from build123d import *

# Parameters (mm, degrees)
IZIM1_W                     = 140
IZIM1_H                     = 65
Y_KSEKLIK_EKSTR_ZYON1_DEPTH = 25
BO_ALTMA3_T                 = 6
IZIM2_R                     = 2.25
KES_EKSTR_ZYON1_DEPTH       = 25
IZIM3_W                     = 13.33242511
IZIM3_H                     = 17.74072696
KES_EKSTR_ZYON2_DEPTH       = 25
RADYUS1_R                   = 2
IZIM2_2_R                   = 2.25
Y_KSEKLIK_EKSTR_ZYON2_DEPTH = 56
IZIM4_W                     = 373.647540747
IZIM4_H                     = 192.392001967
KES_EKSTR_ZYON3_DEPTH       = 1
IZIM5_R                     = 2.25
KES_EKSTR_ZYON4_DEPTH       = 25
IZIM6_W                     = 175.161164464
IZIM6_H                     = 86.760539326
KES_EKSTR_ZYON5_DEPTH       = 37
IZIM7_R                     = 2.25
Y_KSEKLIK_EKSTR_ZYON3_DEPTH = 30
IZIM8_R                     = 1
KES_EKSTR_ZYON6_DEPTH       = 16
KES_EKSTR_ZYON7_START       = -16
IZIM9_R                     = 1
KES_EKSTR_ZYON7_DEPTH       = 16
M2_DI_LI_DELIK2_D           = 1.6
M2_DI_LI_DELIK2_CSINK_D     = 2.05
M2_DI_LI_DELIK2_CSINK_ANGLE = 82
M2_DI_LI_DELIK3_D           = 1.6
M2_DI_LI_DELIK3_CSINK_D     = 2.05
M2_DI_LI_DELIK3_CSINK_ANGLE = 82
IZIM16_W                    = 12
IZIM16_H                    = 6
IZIM16_R                    = 1
Y_KSEKLIK_EKSTR_ZYON4_DEPTH = 2.5
Y_KSEKLIK_EKSTR_ZYON5_START = 2.5
IZIM17_W                    = 12
IZIM17_H                    = 6
IZIM17_R                    = 1
Y_KSEKLIK_EKSTR_ZYON5_DEPTH = 2.5
PAH1_SIZE                   = 2.5


# Read off the part's stored shape, not the designer's step: M2 Dişli Delik4
with BuildPart() as part:
    # Çizim1 → Yükseklik-Ekstrüzyon1 (new body)
    with BuildSketch(Plane.XY):
        Rectangle(IZIM1_W, IZIM1_H)
    extrude(amount=Y_KSEKLIK_EKSTR_ZYON1_DEPTH)

    # İç Boşaltma3
    bo_altma3_openings = [part.faces().sort_by_distance(p)[0] for p in [
        (0, 0, 0),
    ]]
    offset(amount=BO_ALTMA3_T, openings=bo_altma3_openings, kind=Kind.INTERSECTION)

    # Çizim2 → Kes-Ekstrüzyon1 (cut)
    with BuildSketch(Plane(origin=(0, 0, 0), x_dir=(-1, 0, 0), z_dir=(0, 0, -1))):
        with Locations((-73, -35.5)):
            Circle(IZIM2_R)
        with Locations(Location((73, -35.5, 0), (0, 0, 180))):
            Circle(IZIM2_R)
        with Locations(Location((-73, 35.5, 0), (0, 0, 180))):
            Circle(IZIM2_R)
        with Locations((73, 35.5)):
            Circle(IZIM2_R)
    extrude(amount=-KES_EKSTR_ZYON1_DEPTH, mode=Mode.SUBTRACT)

    # Çizim3 → Kes-Ekstrüzyon2 (cut)
    with BuildSketch(Plane.ZY.offset(-70)):
        with Locations((15.822558672, 0)):
            Rectangle(IZIM3_W, IZIM3_H)
    extrude(amount=-KES_EKSTR_ZYON2_DEPTH, mode=Mode.SUBTRACT)

    # Radyus1
    radyus1_edges = [part.edges().sort_by_distance(p)[0] for p in [
        (76, -38.5, 15.5),
        (-76, -38.5, 15.5),
        (-76, 38.5, 15.5),
        (76, 38.5, 15.5),
    ]]
    fillet(radyus1_edges, radius=RADYUS1_R)

    # Çizim2<2> → Yükseklik-Ekstrüzyon2 (add)
    with BuildSketch(Plane(origin=(0, 0, 0), x_dir=(-1, 0, 0), z_dir=(0, 0, -1))):
        with Locations((-73, -35.5)):
            Circle(IZIM2_2_R)
        with Locations((73, -35.5)):
            Circle(IZIM2_2_R)
        with Locations((-73, 35.5)):
            Circle(IZIM2_2_R)
        with Locations((73, 35.5)):
            Circle(IZIM2_2_R)
    extrude(amount=-Y_KSEKLIK_EKSTR_ZYON2_DEPTH)

    # Çizim4 → Kes-Ekstrüzyon3 (cut)
    with BuildSketch(Plane.XY.offset(56)):
        with Locations((-92.221826013, 44.195860188)):
            Rectangle(IZIM4_W, IZIM4_H)
    extrude(amount=-KES_EKSTR_ZYON3_DEPTH, mode=Mode.SUBTRACT)

    # Çizim5 → Kes-Ekstrüzyon4 (cut)
    with BuildSketch(Plane(origin=(0, 0, 0), x_dir=(-1, 0, 0), z_dir=(0, 0, -1))):
        with Locations((-73, -35.527793561)):
            Circle(IZIM5_R)
        with Locations(Location((-73, 35.527793561, 0), (0, 0, 180))):
            Circle(IZIM5_R)
        with Locations((73, 35.527793561)):
            Circle(IZIM5_R)
        with Locations(Location((73, -35.527793561, 0), (0, 0, 180))):
            Circle(IZIM5_R)
    extrude(amount=-KES_EKSTR_ZYON4_DEPTH, mode=Mode.SUBTRACT)

    # Çizim6 → Kes-Ekstrüzyon5 (cut)
    with BuildSketch(Plane.XY.offset(31)):
        Rectangle(IZIM6_W, IZIM6_H)
    extrude(amount=KES_EKSTR_ZYON5_DEPTH, mode=Mode.SUBTRACT)

    # Çizim7 → Yükseklik-Ekstrüzyon3 (add)
    with BuildSketch(Plane(origin=(0, 0, 0), x_dir=(-1, 0, 0), z_dir=(0, 0, -1))):
        with Locations((-73, 35.527793561)):
            Circle(IZIM7_R)
        with Locations((-73, -35.527793561)):
            Circle(IZIM7_R)
        with Locations((73, -35.527793561)):
            Circle(IZIM7_R)
        with Locations((73, 35.527793561)):
            Circle(IZIM7_R)
    extrude(amount=-Y_KSEKLIK_EKSTR_ZYON3_DEPTH)

    # Çizim8 → Kes-Ekstrüzyon6 (cut)
    with BuildSketch(Plane(origin=(76, 0, 0), x_dir=(0, 0, -1), z_dir=(1, 0, 0))):
        with Locations((-3, 28.5)):
            Circle(IZIM8_R)
        with Locations(Location((-3, -28.5, 0), (0, 0, 180))):
            Circle(IZIM8_R)
    extrude(amount=-KES_EKSTR_ZYON6_DEPTH, mode=Mode.SUBTRACT)

    # Çizim9 → Kes-Ekstrüzyon7 (cut)
    with BuildSketch(Plane.ZY.offset(76).offset(KES_EKSTR_ZYON7_START)):
        with Locations(Location((3, 28.5, 0), (0, 0, 180))):
            Circle(IZIM9_R)
        with Locations((3, -28.5)):
            Circle(IZIM9_R)
    extrude(amount=KES_EKSTR_ZYON7_DEPTH, mode=Mode.SUBTRACT)

    # M2 Dişli Delik2 (through all)
    with Locations(Plane(origin=(-76, 28.5, 3), x_dir=(0, 0, -1), z_dir=(-1, 0, 0))):
        with Locations((0, 0), (0, 57)):
            CounterSinkHole(M2_DI_LI_DELIK2_D / 2, M2_DI_LI_DELIK2_CSINK_D / 2, counter_sink_angle=M2_DI_LI_DELIK2_CSINK_ANGLE)

    # M2 Dişli Delik3 (through all)
    with Locations(Plane(origin=(76, 28.5, 3), x_dir=(0, 0, 1), z_dir=(1, 0, 0))):
        with Locations((0, 0), (0, 57)):
            CounterSinkHole(M2_DI_LI_DELIK3_D / 2, M2_DI_LI_DELIK3_CSINK_D / 2, counter_sink_angle=M2_DI_LI_DELIK3_CSINK_ANGLE)

    # Çizim16 → Yükseklik-Ekstrüzyon4 (add)
    # profile 1 of 2: a face of its own
    with BuildSketch(Plane(origin=(76, 0, 0), x_dir=(0, 0, -1), z_dir=(1, 0, 0))):
        with Locations((-31, 28.5)):
            Rectangle(IZIM16_W, IZIM16_H)
        with Locations((-34, 28.5)):
            Circle(IZIM16_R, mode=Mode.SUBTRACT)
    # profile 2 of 2: a face of its own
    with BuildSketch(Plane(origin=(76, 0, 0), x_dir=(0, 0, -1), z_dir=(1, 0, 0))):
        with Locations((-31, -28.5)):
            Rectangle(IZIM16_W, IZIM16_H)
        with Locations(Location((-34, -28.5, 0), (0, 0, 180))):
            Circle(IZIM16_R, mode=Mode.SUBTRACT)
    extrude(amount=Y_KSEKLIK_EKSTR_ZYON4_DEPTH)

    # Çizim17 → Yükseklik-Ekstrüzyon5 (add)
    # profile 1 of 2: a face of its own
    with BuildSketch(Plane.ZY.offset(76).offset(Y_KSEKLIK_EKSTR_ZYON5_START)):
        with Locations((31, 28.5)):
            Rectangle(IZIM17_W, IZIM17_H)
        with Locations(Location((34, 28.5, 0), (0, 0, 180))):
            Circle(IZIM17_R, mode=Mode.SUBTRACT)
    # profile 2 of 2: a face of its own
    with BuildSketch(Plane.ZY.offset(76).offset(Y_KSEKLIK_EKSTR_ZYON5_START)):
        with Locations((31, -28.5)):
            Rectangle(IZIM17_W, IZIM17_H)
        with Locations((34, -28.5)):
            Circle(IZIM17_R, mode=Mode.SUBTRACT)
    extrude(amount=-Y_KSEKLIK_EKSTR_ZYON5_DEPTH)

    # M2 Dişli Delik4 outline → M2 Dişli Delik4 (revolve, cut)
    with BuildSketch(Plane(origin=(0, 28.5, 34), x_dir=(0, 1, 0), z_dir=(0, 0, -1))):
        Polygon((1, 78.5), (1, 78.47124079), (1.025, 78.5), align=None)
        Polygon((1.025, -78.5), (1, -78.47124079), (1, -78.5), align=None)
    revolve(axis=Axis((0, 28.5, 34), (1, 0, 0)), mode=Mode.SUBTRACT)

    # M2 Di_li Delik4 2 outline → M2 Di_li Delik4 2 (revolve, cut)
    with BuildSketch(Plane(origin=(0, -28.5, 34), x_dir=(0, 1, 0), z_dir=(0, 0, -1))):
        Polygon((1, 78.5), (1, 78.47124079), (1.025, 78.5), align=None)
        Polygon((1.025, -78.5), (1, -78.47124079), (1, -78.5), align=None)
    revolve(axis=Axis((0, -28.5, 34), (1, 0, 0)), mode=Mode.SUBTRACT)

    # Pah1
    pah1_edges = [part.edges().sort_by_distance(p)[0] for p in [
        (76, -28.5, 25),
        (76, 28.5, 25),
        (-76, 28.5, 25),
        (-76, -28.5, 25),
    ]]
    chamfer(pah1_edges, length=PAH1_SIZE - 0.0001)  # a hair under: the kernel refuses the full size


solid = part.part
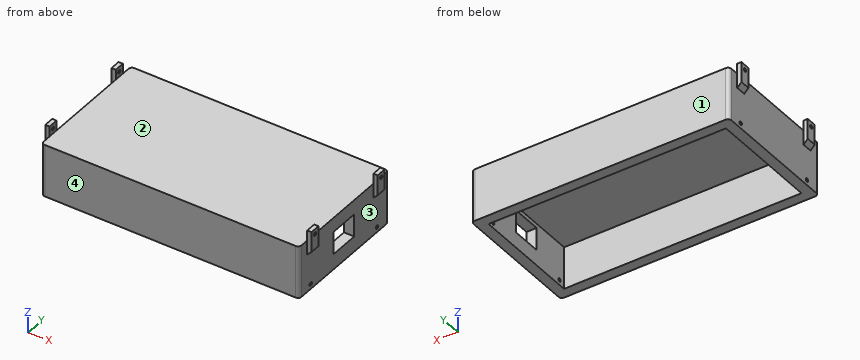
Read the model definition and answer for the solid it produces. Units are mm, in the model's axes. Face numbers are marked on the shaded views. Round coordinates to 2 decimals unless told otherwise and drop trailing zeros. Loops run counter-clockwise (first coordinate to the right, second up) from the corner with the lowest first, then second, coordinate; pieces in that order, holes last.
Q1. Section D-D on y = 14 is taken. Write down the section's boundary in (x, z), and give its area (3 significant figures).
Q2. Each of these flat-tipped pins is pushed along its axis until it touches: pin 1 (9.5 mm diameter, centred on y = 18, z = 11.5, fed in from -X); pin 2 (4 mm diameter, centred on x = -8.5, y = -6, fed in from +Z); pin 3 (3 mm diameter, centred on x = -77.5, z = 32.5, fed in from +Y). Where does it stop, or does it pass through?
Q3. Consider probe 1 along Y at (x, z) = (-73.05, 3); probe 2 along Y at (x, z) = (-76.55, 34); probe 3 along Y at (x, z) = (-31, 11.5). Determine where each line is inside the solid, lowest interval first.
Q4. Section B-B on z = 28.5 is taken. Write down the section's boundary in (x, y).
Q5. Section C-C on x = -43 is taken. Write down the section's boundary in (y, z), and give its area (3 significant figures).
Q6. Section A-A on y = 5.5 is taken. Write down the section's boundary in (x, z), and give its area (3 significant figures).
Q7. Determine the mould class of the marked faces 1, 2, 3 and 4 for opening direction Y: released by +Y, released by -Y, zero draft, split by the parting line, or undercut.
Output:
1. outline: (-76, 0) - (-70, 0) - (-70, 25) - (70, 25) - (70, 0) - (76, 0) - (76, 31) - (-76, 31) - close
1. area: 1,210 mm2
2. pin 1: stops at x = -76
2. pin 2: stops at z = 31
2. pin 3: stops at y = 31.5
3. probe 1: y = -38.5 to -29.5, -27.5 to 27.5, 29.5 to 38.5
3. probe 2: y = -31.5 to -29.5, -27.5 to -25.5, 25.5 to 27.5, 29.5 to 31.5
3. probe 3: y = -38.5 to -32.5, 32.5 to 38.5
4. outline: (-78.5, -31.5) - (-76, -31.5) - (-76, -36.5) arc R2 ccw to (-74, -38.5) - (74, -38.5) arc R2 ccw to (76, -36.5) - (76, -31.5) - (78.5, -31.5) - (78.5, -25.5) - (76, -25.5) - (76, 25.5) - (78.5, 25.5) - (78.5, 31.5) - (76, 31.5) - (76, 36.5) arc R2 ccw to (74, 38.5) - (-74, 38.5) arc R2 ccw to (-76, 36.5) - (-76, 31.5) - (-78.5, 31.5) - (-78.5, 25.5) - (-76, 25.5) - (-76, -25.5) - (-78.5, -25.5) - close
5. outline: (-38.5, 0) - (-32.5, 0) - (-32.5, 25) - (32.5, 25) - (32.5, 0) - (38.5, 0) - (38.5, 31) - (-38.5, 31) - close
5. area: 762 mm2
6. outline: (-76, 0) - (-70, 0) - (-70, 25) - (70, 25) - (70, 22.49) - (76, 22.49) - (76, 31) - (-76, 31) - close; (70, 0) - (76, 0) - (76, 9.16) - (70, 9.16) - close
6. area: 1,130 mm2
7. face 1: released by +Y
7. face 2: zero draft
7. face 3: undercut
7. face 4: released by -Y
